from build123d import *

# Parameters (mm, degrees)
BOSS_EXTRUDE1_DEPTH = 72
SKETCH3_R           = 6
CUT_EXTRUDE1_DEPTH  = 72


with BuildPart() as part:
    # Sketch1 → Boss-Extrude1 (new body)
    with BuildSketch(Plane.XY):
        Polygon((0, 0), (0, 10), (35, 10), (35, 13), (85, 13), (85, 10), (120, 10), (120, 0), (88, 0), (83.349169446, 4.650830554), (36.650830554, 4.650830554), (32, 0), align=None)
    extrude(amount=BOSS_EXTRUDE1_DEPTH)

    # Sketch3 → Cut-Extrude1 (cut)
    with BuildSketch(Plane(origin=(0, 10, 0), x_dir=(1, 0, 0), z_dir=(0, 1, 0))):
        with Locations(Location((12, -12, 0), (0, 0, 270))):
            Circle(SKETCH3_R)
        with Locations(Location((108, -12, 0), (0, 0, 270))):
            Circle(SKETCH3_R)
        with Locations(Location((108, -60, 0), (0, 0, 270))):
            Circle(SKETCH3_R)
        with Locations(Location((12, -60, 0), (0, 0, 270))):
            Circle(SKETCH3_R)
        with BuildLine():
            ThreePointArc((0, -12), (3.514718626, -3.514718626), (12, 0))
            Line((12, 0), (0, 0))
            Line((0, 0), (0, -12))
        make_face()
        with BuildLine():
            ThreePointArc((12, -72), (3.514718626, -68.485281374), (0, -60))
            Line((0, -60), (0, -72))
            Line((0, -72), (12, -72))
        make_face()
        with BuildLine():
            Line((120, -72), (120, -60))
            ThreePointArc((120, -60), (116.485281374, -68.485281374), (108, -72))
            Line((108, -72), (120, -72))
        make_face()
        with BuildLine():
            Line((120, 0), (108, 0))
            ThreePointArc((108, 0), (116.485281374, -3.514718626), (120, -12))
            Line((120, -12), (120, 0))
        make_face()
    extrude(amount=-CUT_EXTRUDE1_DEPTH, mode=Mode.SUBTRACT)


solid = part.part
Part model, mm, in its own coordinate system. A direction names the side the tool comes from. Coordinates: 2 decimals unless noted, no trailing zeros. Write each loop counter-clockwise with the first axis right and the second up, starting at its lowest first coordinate (ties: lowest second). Pieces come first, ordered by that corner, then holes. Notation, with made-up numbers: (66.25, 75.25) - (79.25, 75.25) arc R22 ccw to (79.25, 108.25) - close; hole circle Ø3 at (9, 35). An arc over 180 degrees is marked (long way). Put each result on its own line as item: value.
1. Probe line 1 along X through (y, z) = (3, 60); line 2 along X through (y, z) = (5, 12); line 3 along X through (y, z) = (2.5, 12). List the from-to ranges inside material, lowest first. Write a range as [from, to].
Final values:
line 1: x = [0, 6], [18, 35], [85, 102], [114, 120]
line 2: x = [0, 6], [18, 102], [114, 120]
line 3: x = [0, 6], [18, 34.5], [85.5, 102], [114, 120]
2. Band-saw the part on C-C (x = 16.5). Write the cut outline in (y, z).
Final values:
outline: (0, 0) - (10, 0) - (10, 8.03) - (0, 8.03) - close; (0, 15.97) - (10, 15.97) - (10, 56.03) - (0, 56.03) - close; (0, 63.97) - (10, 63.97) - (10, 72) - (0, 72) - close
3. 3-axis set-ups, long thin cutter, end or side, ignore diameter. For faces 4 (the cylindrical face through (12, 5, 54)), 5 (the flat face through (85, 12, 35)), 6 (the flat face through (60, 4.651, 35)): which of +Z, -Z, +X, -X, +Y, -Y reach the whole face in a straight line?
Final values:
face 4: +Y, -Y
face 5: +Z, -Z, +X, +Y
face 6: +Z, -Z, -Y
4. Band-saw the part on D-D (z = 48). Write the cut outline in (x, y).
Final values:
outline: (0, 0) - (32, 0) - (36.65, 4.65) - (83.35, 4.65) - (88, 0) - (120, 0) - (120, 10) - (85, 10) - (85, 13) - (35, 13) - (35, 10) - (0, 10) - close
5. Flat gauge pins, fed straight in: pin 1 Ø2.5 at (y, z) = (12, 50) entering from -X; pin 2 Ø9.5 at (x, z) = (12, 12) entering from -Y; pin 3 Ø3 at (y, z) = (8.5, 7.5) entering from -X; pin 4 Ø1.5 at (y, z) = (11, 26.5) entering from +X. Where does each tip first touch, or does it go through?
Final values:
pin 1: stops at x = 35
pin 2: passes through
pin 3: stops at x = 0.38
pin 4: stops at x = 85
6. Band-saw the part on B-B (z = 15.5). Write the cut outline in (x, y).
Final values:
outline: (0, 0) - (7.13, 0) - (7.13, 10) - (0, 10) - close; (16.87, 0) - (32, 0) - (36.65, 4.65) - (83.35, 4.65) - (88, 0) - (103.13, 0) - (103.13, 10) - (85, 10) - (85, 13) - (35, 13) - (35, 10) - (16.87, 10) - close; (112.87, 0) - (120, 0) - (120, 10) - (112.87, 10) - close
7. Band-saw the part on A-A (y = 7.25). Write the cut outline in (x, z).
Final values:
outline: (0, 12) arc R12 ccw to (12, 0) - (108, 0) arc R12 ccw to (120, 12) - (120, 60) arc R12 ccw to (108, 72) - (12, 72) arc R12 ccw to (0, 60) - close; hole circle Ø12 at (12, 12); hole circle Ø12 at (12, 60); hole circle Ø12 at (108, 12); hole circle Ø12 at (108, 60)
8. Two-plate mould, pull along X, no slides. Class faces 1 (the flat face through (0, 5, 36)), 2 (the flat face through (102, 10, 35)), 3 (the flat face through (34, 2, 35)): +X half, -X half, draft (parallel to the pull), parting line (faces both ways), or undercut.
Final values:
face 1: -X half
face 2: draft
face 3: undercut
